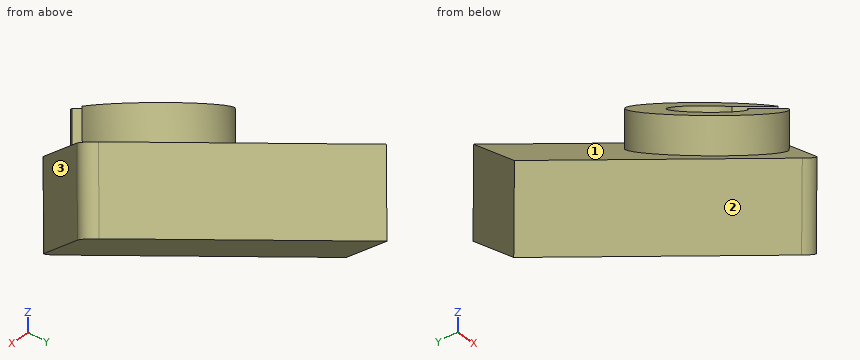
```python
from build123d import *

# Parameters (mm, degrees)
F1_DEPTH = 106
F2_DEPTH = 150
F3_ANGLE = 30
F4_ANGLE = 30
F5_ANGLE = 30


with BuildPart() as f1:
    # F0 (on Top) → F1 (new body)
    with BuildSketch(Plane.XY):
        with BuildLine():
            Line((340, 185), (20, 185))
            Line((20, 185), (20, -40))
            Line((20, -40), (340, -40))
            ThreePointArc((340, -40), (354.1421356237, -34.1421356237), (360, -20))
            Line((360, -20), (360, 165))
            ThreePointArc((360, 165), (354.1421356237, 179.1421356237), (340, 185))
        make_face()
        with BuildLine():
            ThreePointArc((350, 90), (171.2961296312, 74.7808219147), (344.8528137424, 120))
            Line((344.8528137424, 120), (293.5410196625, 120))
            ThreePointArc((293.5410196625, 120), (217.9622438467, 73.9430059602), (305, 90))
            Line((305, 90), (350, 90))
        make_face(mode=Mode.SUBTRACT)
        with BuildLine():
            Line((293.5410196625, 120), (344.8528137424, 120))
            ThreePointArc((344.8528137424, 120), (171.2961296312, 74.7808219147), (350, 90))
            Line((350, 90), (305, 90))
            ThreePointArc((305, 90), (217.9622438467, 73.9430059602), (293.5410196625, 120))
        make_face()
    extrude(amount=F1_DEPTH)

    # F0 (on Top) → F2 (join)
    with BuildSketch(Plane.XY):
        with BuildLine():
            Line((293.5410196625, 120), (344.8528137424, 120))
            ThreePointArc((344.8528137424, 120), (171.2961296312, 74.7808219147), (350, 90))
            Line((350, 90), (305, 90))
            ThreePointArc((305, 90), (217.9622438467, 73.9430059602), (293.5410196625, 120))
        make_face()
    extrude(amount=F2_DEPTH)


with BuildPart() as f1_1:
    # F3: moved
    add(f1.part.rotate(Axis((180, -40, 0), (1, 0, 0)), F3_ANGLE))


with BuildPart() as f1_2:
    # F4: moved
    add(f1_1.part.rotate(Axis((20, 4.4278579257, 148.0486928012), (0, -0.8660254038, -0.5)), F4_ANGLE))


with BuildPart() as f1_3:
    # F5: moved
    add(f1_2.part.rotate(Axis((46.5, -70.0503267997, 52.0486928012), (0.5, 0.4330127019, -0.75)), F5_ANGLE))


solid = f1_3.part
```
Check sheet for the modelled part. Datum: model origin and axes. Units: mm. Face numbers are marked on the shaded views. Round coordinates to 2 decimals unless told otherwise and drop trailing zeros. Loops run counter-clockwise (first coordinate to the right, second up) from the corner with the lowest first, then second, coordinate; pieces in that order, holes last. Notation, with made-up numbers: (0.5, 22) - (27.5, 22) arc R5 ccw to (27.5, 28) - close; hole circle Ø11 at (30, -28.5). An arc over 180 degrees is marked (long way). Write item = value, one per line. Start each with the question number.
Q1. Section check A-A (y = -55.5). Record the boundary of the cut face in (x, z), plus the area to 3 significant figures.
Q2. Section check B-B (x = 144.5). Record the boundary of the cut face in (y, z), plus the area to 3 significant figures.
Q3. Section check C-C (y = 8.5). Record the boundary of the cut face in (x, z).
Q4. Depth check by flat-ended pin: P1, Ø5, axis at y = -215.5, z = 138.5, coming from the -X side; P2, Ø6, axis at x = 245, y = -203.5, coming from the -Z side; P3, Ø2, axis at x = 227, z = 255, coming from the +Y side. Enter the tip coordinate at first touch or a pass-through.
Q5. Thickness scan on L1, parallel to Z at x = 145, y = -49; L2, parallel to X at y = -46, z = 187; L3, parallel to X at y = -177, z = 80. Record the ranges inside material, lowest first.
Q6. Release check for a two-part mould opening along Z. For the marked faces 1, 2 and 3 record: pulls with the +Z half, pulls with the -Z half, needs draft (parallel to the pull), parting line crosses it, or undercut.
Derived:
q1.outline = (45.98, 130.77) - (63.3, 26.85) - (82.7, 13.92) - (342.51, 187.12) - (236.51, 257.79) - close
q1.area = 32,700 mm^2
q2.outline = (-200.82, 112.55) - (-109.02, 24.22) - (56.1, 119.55) - (71.07, 197.33) - (24.18, 242.45) - close
q2.area = 29,700 mm^2
q3.outline = (90.32, 197.28) - (111.52, 70.08) - (268.61, 174.8) - (162.61, 245.47) - close
q4.P1 = 191.81
q4.P2 = 44.62
q4.P3 = -44.77
q5.L1 = 59.2 to 200.54
q5.L2 = 122.1 to 328.97
q5.L3 = 158.94 to 287.05
q6.face_1 = undercut
q6.face_2 = pulls with the -Z half
q6.face_3 = pulls with the +Z half
